```python
from build123d import *

# Parameters (mm, degrees)
EXTRUDE_1_DEPTH     = 16
SKETCH_3_W          = 16
SKETCH_3_H          = 4.26667426
EXTRUDE_3_DEPTH     = 16
SKETCH_23_W         = 16
SKETCH_23_H         = 4.26667426
EXTRUDE_4_DEPTH     = 16
F_2_0MM_2_D         = 2.6
F_2_0MM_3_D         = 2.6
SKETCH_33_W         = 45.5
SKETCH_33_H         = 16
EXTRUDE_5_DEPTH     = 1
SKETCH_34_W         = 28.538779463
SKETCH_34_H         = 11.2
EXTRUDE_6_DEPTH     = 20
CUT_EXTRUDE_1_DEPTH = 20


with BuildPart() as part:
    # 草图2 → 凸台-拉伸1 (new body)
    with BuildSketch(Plane.XY):
        Polygon((34.591799544, 12.66332574), (-20.108200456, 12.66332574), (-20.108200456, -4.26667426), (-15.508200456, -4.26667426), (-15.508200456, 8.06332574), (29.991799544, 8.06332574), (29.991799544, -4.26667426), (34.591799544, -4.26667426), align=None)
    extrude(amount=EXTRUDE_1_DEPTH)

    # 草图3 → 凸台-拉伸3 (add)
    with BuildSketch(Plane.ZY.offset(20.108200456)):
        with Locations((8, -2.13333713)):
            Rectangle(SKETCH_3_W, SKETCH_3_H)
    extrude(amount=EXTRUDE_3_DEPTH)

    # 草图23 → 凸台-拉伸4 (add)
    with BuildSketch(Plane(origin=(34.591799544, 0, 0), x_dir=(0, 0, -1), z_dir=(1, 0, 0))):
        with Locations((-8, -2.13333713)):
            Rectangle(SKETCH_23_W, SKETCH_23_H)
    extrude(amount=EXTRUDE_4_DEPTH)

    # Ø2.0mm 暗销孔2 (through all)
    with Locations(Plane(origin=(0, 0, 0), x_dir=(1, 0, 0), z_dir=(0, 1, 0))):
        with Locations((42.591799544, -8)):
            Hole(F_2_0MM_2_D / 2)

    # Ø2.0mm 暗销孔3 (through all)
    with Locations(Plane(origin=(0, 0, 0), x_dir=(1, 0, 0), z_dir=(0, 1, 0))):
        with Locations((-28.108200456, -8)):
            Hole(F_2_0MM_3_D / 2)

    # 草图33 → 凸台-拉伸5 (add)
    with BuildSketch(Plane.XZ.offset(-8.06332574)):
        with Locations((7.241799544, 8)):
            Rectangle(SKETCH_33_W, SKETCH_33_H)
    extrude(amount=EXTRUDE_5_DEPTH)

    # 草图34 → 凸台-拉伸6 (add)
    with BuildSketch(Plane(origin=(0, 12.66332574, 0), x_dir=(1, 0, 0), z_dir=(0, 1, 0))):
        with Locations((-5.838810725, -8)):
            Rectangle(SKETCH_34_W, SKETCH_34_H)
    extrude(amount=EXTRUDE_6_DEPTH)

    # 草图35 → 切除-拉伸1 (cut)
    with BuildSketch(Plane.XY.offset(16)):
        Polygon((-3.808200456, 12.66332574), (2.116069444, 32.66332574), (-2.683930556, 32.66332574), (-8.608200456, 12.66332574), align=None)
        Polygon((-1.808200456, 12.66332574), (8.430579007, 12.66332574), (8.430579007, 32.66332574), (4.116069444, 32.66332574), align=None)
        Polygon((-20.108200456, 12.66332574), (-10.608200456, 12.66332574), (-4.683930556, 32.66332574), (-20.108200456, 32.66332574), align=None)
    extrude(amount=-CUT_EXTRUDE_1_DEPTH, mode=Mode.SUBTRACT)


solid = part.part
```
The model under review builds one solid part; all positions refer to its coordinate system, in mm. A direction names the side the tool comes from. Round coordinates to 2 decimals unless told otherwise and drop trailing zeros. Loops run counter-clockwise (first coordinate to the right, second up) from the corner with the lowest first, then second, coordinate; pieces in that order, holes last. Notation, with made-up numbers: (-10, 19) - (22, 19) arc R21 cw to (22, 49) - close; hole circle Ø4 at (-16.5, 85). An arc over 180 degrees is marked (long way). Use a Markdown table: item, result. Add a question column.
Q1. Add section A-A (y = 14). State the section outline as (x, z) points.
Q2. Add section D-D (x = 27). State the section outline as (y, z) points, plus the area to 3 significant figures.
Q3. Insertion check: pin 1 Ø1.5 at (y, z) = (3.5, 9.5) entering from -X; pin 2 Ø2.5 at (x, y) = (-5, 26.5) entering from +Z; pin 3 Ø2.5 at (x, y) = (-5, 26.5) entering from -Z. Each pin has a flat end and moves straight along its axis. Give the tip position at first contact, or say it passes through.
Q4. For probe 1 along X at (y, z) = (-1.2, 8); probe 2 along X at (y, z) = (1.5, 6.5); probe 3 along X at (y, z) = (-2, 8.5), list the stretches that pass through material, from the lowest coordinate up.
Q5. Add section B-B (x = 0). State the section outline as (y, z) points.
Q6. The part is to be moulded in two halves that separate along X. For faces 5 (the face through (-20.108, 6, 8)), 6 (the face through (-4, 32.663, 8)), 7 (the face through (7, 7.063, 8)), 8 (the face through (-0.89, 22.52, 8.08)), say which applies: pulls with the +X half, pulls with the -X half, needs draft (parallel to the pull), parting line crosses it, or undercut.
Q7. Machinability: for faces 1 (the face through (42, 0, 10)), 2 (the face through (29.992, 1, 8)), 3 (the face through (1.195, 22.803, 8.078)), 4 (the face through (0, 23, 13.6)), which of the approach directions +Z, -Z, +X, -X, +Y, -Y give a long, thin tool a straight path to every point of the face, cutting with its end or side? Answer none if there is none.
Q8. Add section C-C (z = 4.5). State the section outline as (x, y) points, plus the area to 3 significant figures.
Worked answers:
| question | item | result |
|---|---|---|
| 1 | outline | (-10.21, 2.4) - (-8.21, 2.4) - (-8.21, 13.6) - (-10.21, 13.6) - close; (-3.41, 2.4) - (-1.41, 2.4) - (-1.41, 13.6) - (-3.41, 13.6) - close |
| 2 | outline | (7.06, 0) - (12.66, 0) - (12.66, 16) - (7.06, 16) - close |
| 2 | area | 89.6 mm² |
| 3 | pin 1 | x = -20.11 |
| 3 | pin 2 | z = 13.6 |
| 3 | pin 3 | z = 2.4 |
| 4 | probe 1 | -36.11 to -29.41, -26.81 to -15.51, 29.99 to 41.29, 43.89 to 50.59 |
| 4 | probe 2 | -20.11 to -15.51, 29.99 to 34.59 |
| 4 | probe 3 | -36.11 to -29.31, -26.91 to -15.51, 29.99 to 41.39, 43.79 to 50.59 |
| 5 | outline | (7.06, 0) - (12.66, 0) - (12.66, 16) - (7.06, 16) - close; (18.77, 2.4) - (25.52, 2.4) - (25.52, 13.6) - (18.77, 13.6) - close |
| 6 | face 5 | pulls with the -X half |
| 6 | face 6 | needs draft |
| 6 | face 7 | undercut |
| 6 | face 8 | undercut |
| 7 | face 1 | +Z, -Z, +X, +Y |
| 7 | face 2 | +Z, -Z, -Y |
| 7 | face 3 | +Z, -Z, +X |
| 7 | face 4 | +Z, +X, -X, +Y |
| 8 | outline | (-36.11, -4.27) - (-15.51, -4.27) - (-15.51, 7.06) - (29.99, 7.06) - (29.99, -4.27) - (50.59, -4.27) - (50.59, 0) - (34.59, 0) - (34.59, 12.66) - (-1.81, 12.66) - (4.12, 32.66) - (2.12, 32.66) - (-3.81, 12.66) - (-8.61, 12.66) - (-2.68, 32.66) - (-4.68, 32.66) - (-10.61, 12.66) - (-20.11, 12.66) - (-20.11, 0) - (-36.11, 0) - close |
| 8 | area | 627 mm² |
